Read the model definition and answer for the solid it produces. Units are mm, in the model's axes. Give positions to 0.01 mm unless a question says otherwise; leave off trailing zeros. Order: outer loops, then holes, each group sorted by start corner. A loop starts at its lowest first (then second) coordinate and runs counter-clockwise, first axis right, second up.
Item 1: A cutting plane is placed at C-C (z = 146). Write down the section's boundary in (x, y).
Item 2: A cutting plane is placed at B-B (y = 3.3). State how many separate pieces and enclosed holes the cut face has, plus the area to 3 significant figures.
Item 3: A cutting plane is placed at A-A (z = 9). Write down the section's boundary in (x, y), plus the area to 3 significant figures.
Item 4: Find the intervals of material crossed by line 1 along X through (y, z) = (1.1, 92.08); line 2 along Z through (x, y) = (-95.1, 4.05); line 3 along Z through (x, y) = (-94, 2), in increasing order.
Item 5: Given pin 1 Ø2.5 at (x, y) = (130.5, 3) entering from -Z; pin 2 Ø1.2 at (x, y) = (-107, 3) entering from -Z; pin 3 Ø1 at (y, z) = (3, 145.5) entering from +X, each flat-ended and moving along its own axis, determine where each tip first touches the part or whether it passes through.
from build123d import *

# Parameters (mm, degrees)
ESQUISSE1_W              = 280.2
ESQUISSE1_H              = 276.282873123
BOSS_EXTRU_1_DEPTH       = 5
ENL_V_MAT_EXTRU_3_DEPTH  = 283.344868376
ENL_V_MAT_EXTRU_5_DEPTH  = 283.344868376
ESQUISSE8_R              = 1.5
ENL_V_MAT_EXTRU_8_DEPTH  = 283.344868376
ENL_V_MAT_EXTRU_15_DEPTH = 283.344868376
CONG_1_R                 = 10
ESQUISSE13_R             = 1.5
ENL_V_MAT_EXTRU_16_DEPTH = 220.422993326
ESQUISSE14_R             = 1.6
ENL_V_MAT_EXTRU_17_DEPTH = 220.422993326


with BuildPart() as part:
    # Esquisse1 → Boss.-Extru.1 (new body)
    with BuildSketch(Plane(origin=(0, 0, 0), x_dir=(1, 0, 0), z_dir=(0, 1, 0))):
        with Locations((0, -106.941436562)):
            Rectangle(ESQUISSE1_W, ESQUISSE1_H)
    extrude(amount=BOSS_EXTRU_1_DEPTH)

    # Esquisse4 → Enlèv. mat.-Extru.3 (cut, through all)
    with BuildSketch(Plane(origin=(0, 5, 0), x_dir=(1, 0, 0), z_dir=(0, 1, 0))):
        with BuildLine():
            Line((140.1, -245.082873123), (101.1, -245.082873123))
            ThreePointArc((101.1, -245.082873123), (128.677164466, -233.660037589), (140.1, -206.082873123))
            Line((140.1, -206.082873123), (140.1, -245.082873123))
        make_face()
        with BuildLine():
            Line((-101.1, -245.082873123), (-140.1, -245.082873123))
            Line((-140.1, -245.082873123), (-140.1, -206.082873123))
            ThreePointArc((-140.1, -206.082873123), (-128.677164466, -233.660037589), (-101.1, -245.082873123))
        make_face()
    extrude(amount=-ENL_V_MAT_EXTRU_3_DEPTH, mode=Mode.SUBTRACT)

    # Esquisse6 → Enlèv. mat.-Extru.5 (cut, through all)
    with BuildSketch(Plane(origin=(0, 5, 0), x_dir=(1, 0, 0), z_dir=(0, 1, 0))):
        with BuildLine():
            Line((140.1, 31.2), (53.5, 31.2))
            Line((53.5, 31.2), (53.5, -14))
            ThreePointArc((53.5, -14), (54.964466094, -17.535533906), (58.5, -19))
            Line((58.5, -19), (94.5, -19))
            ThreePointArc((94.5, -19), (98.035533906, -20.464466094), (99.5, -24))
            Line((99.5, -24), (99.5, -28.25))
            ThreePointArc((99.5, -28.25), (100.964466094, -31.785533906), (104.5, -33.25))
            Line((104.5, -33.25), (108.5, -33.25))
            ThreePointArc((108.5, -33.25), (112.035533906, -31.785533906), (113.5, -28.25))
            Line((113.5, -28.25), (113.5, -21.2))
            Line((113.5, -21.2), (123.5, -21.2))
            Line((123.5, -21.2), (123.5, -31.25))
            ThreePointArc((123.5, -31.25), (124.964466094, -34.785533906), (128.5, -36.25))
            Line((128.5, -36.25), (135.1, -36.25))
            ThreePointArc((135.1, -36.25), (138.635533906, -37.714466094), (140.1, -41.25))
            Line((140.1, -41.25), (140.1, 31.2))
        make_face()
        with BuildLine():
            Line((-53.5, -14), (-53.5, 31.2))
            Line((-53.5, 31.2), (-140.1, 31.2))
            Line((-140.1, 31.2), (-140.1, -41.25))
            ThreePointArc((-140.1, -41.25), (-138.635533906, -37.714466094), (-135.1, -36.25))
            Line((-135.1, -36.25), (-128.5, -36.25))
            ThreePointArc((-128.5, -36.25), (-124.964466094, -34.785533906), (-123.5, -31.25))
            Line((-123.5, -31.25), (-123.5, -21.2))
            Line((-123.5, -21.2), (-113.5, -21.2))
            Line((-113.5, -21.2), (-113.5, -28.25))
            ThreePointArc((-113.5, -28.25), (-112.035533906, -31.785533906), (-108.5, -33.25))
            Line((-108.5, -33.25), (-104.5, -33.25))
            ThreePointArc((-104.5, -33.25), (-100.964466094, -31.785533906), (-99.5, -28.25))
            Line((-99.5, -28.25), (-99.5, -24))
            ThreePointArc((-99.5, -24), (-98.035533906, -20.464466094), (-94.5, -19))
            Line((-94.5, -19), (-58.5, -19))
            ThreePointArc((-58.5, -19), (-54.964466094, -17.535533906), (-53.5, -14))
        make_face()
    extrude(amount=-ENL_V_MAT_EXTRU_5_DEPTH, mode=Mode.SUBTRACT)

    # Esquisse8 → Enlèv. mat.-Extru.8 (cut, through all)
    with BuildSketch(Plane.XZ):
        with Locations(Location((-48.5, -26.2, 0), (0, 0, 270))):
            Circle(ESQUISSE8_R)
        with Locations(Location((48.5, -26.2, 0), (0, 0, 270))):
            Circle(ESQUISSE8_R)
    extrude(amount=-ENL_V_MAT_EXTRU_8_DEPTH, mode=Mode.SUBTRACT)

    # Esquisse12 → Enlèv. mat.-Extru.15 (cut, through all)
    with BuildSketch(Plane(origin=(0, 5, 0), x_dir=(1, 0, 0), z_dir=(0, 1, 0))):
        Polygon((-140.1, -96.25), (-75, -168.8), (75, -168.8), (140.1, -96.25), (146.03275504, -294.983631094), (-140.1, -294.983631094), align=None)
    extrude(amount=-ENL_V_MAT_EXTRU_15_DEPTH, mode=Mode.SUBTRACT)

    # Congé1
    cong_1_edges = [part.edges().sort_by_distance(p)[0] for p in [
        (-75, 2.5, 168.8),
        (75, 2.5, 168.8),
    ]]
    fillet(cong_1_edges, radius=CONG_1_R)

    # Esquisse13 → Enlèv. mat.-Extru.16 (cut, through all)
    with BuildSketch(Plane(origin=(0, 5, 0), x_dir=(1, 0, 0), z_dir=(0, 1, 0))):
        with Locations(Location((0.38736006, -154.8, 0), (0, 0, 270))):
            Circle(ESQUISSE13_R)
    extrude(amount=-ENL_V_MAT_EXTRU_16_DEPTH, mode=Mode.SUBTRACT)

    # Esquisse14 → Enlèv. mat.-Extru.17 (cut, through all)
    with BuildSketch(Plane(origin=(0, 5, 0), x_dir=(1, 0, 0), z_dir=(0, 1, 0))):
        with Locations(Location((-95.1, -133.8, 0), (0, 0, 270))):
            Circle(ESQUISSE14_R)
        with Locations(Location((-53.38, -133.8, 0), (0, 0, 270))):
            Circle(ESQUISSE14_R)
        with Locations(Location((-95.1, -92.08, 0), (0, 0, 270))):
            Circle(ESQUISSE14_R)
        with Locations(Location((-53.38, -92.08, 0), (0, 0, 270))):
            Circle(ESQUISSE14_R)
    extrude(amount=-ENL_V_MAT_EXTRU_17_DEPTH, mode=Mode.SUBTRACT)


solid = part.part
Response values:
1. outline: (-95.46, 0) - (95.46, 0) - (95.46, 5) - (-95.46, 5) - close
2. separate pieces: 1
2. enclosed holes: 7
2. area: 41,600 mm2
3. outline: (-53.5, 0) - (53.5, 0) - (53.5, 5) - (-53.5, 5) - close
3. area: 535 mm2
4. line 1: x = -140.1 to -96.7, -93.5 to -54.98, -51.78 to 140.1
4. line 2: z = 19.04 to 90.48, 93.68 to 132.2, 135.4 to 146.4
4. line 3: z = 19 to 90.92, 93.24 to 132.64, 134.96 to 147.63
5. pin 1: stops at z = 36.25
5. pin 2: stops at z = 33.25
5. pin 3: stops at x = 96.36
